Verification items for the finished model (mm, model axes). Face numbers are marked on the shaded views. A direction names the side the tool comes from. Round coordinates to 2 decimals unless told otherwise and drop trailing zeros. Write each loop counter-clockwise with the first axis right and the second up, starting at its lowest first coordinate (ties: lowest second). Pieces come first, ordered by that corner, then holes. Notation, with made-up numbers: (9.25, 83.5) - (44.25, 83.5) arc R19 ccw to (44.25, 110.5) - close; hole circle Ø3 at (43.5, 21.25). An arc over 180 degrees is marked (long way). Answer as a JSON object with one key per item and string values.
```python
from build123d import *

# Parameters (mm, degrees)
CROQUIS1_W                 = 132
CROQUIS1_H                 = 68
SALIENTE_EXTRUIR1_DEPTH    = 8
CORTAR_EXTRUIR1_DEPTH      = 8
CROQUIS3_W                 = 6
CROQUIS3_H                 = 5
SALIENTE_EXTRUIR2_DEPTH    = 8
CROQUIS4_R                 = 2
CROQUIS4_R_2               = 1.6
CORTAR_EXTRUIR2_DEPTH      = 85.029980381
CROQUIS5_R                 = 2.05
CORTAR_EXTRUIR3_DEPTH      = 6
CROQUIS6_W                 = 5
CROQUIS6_H                 = 10
SALIENTE_EXTRUIR3_DEPTH    = 10
CORTAR_EXTRUIR4_DEPTH      = 136.614342899
CORTAR_EXTRUIR4_DEPTH_BACK = 136.614342899
CROQUIS7_R                 = 1.55


with BuildPart() as part:
    # Croquis1 → Saliente-Extruir1 (new body)
    with BuildSketch(Plane(origin=(0, 0, 0), x_dir=(1, 0, 0), z_dir=(0, 1, 0))):
        Rectangle(CROQUIS1_W, CROQUIS1_H)
    extrude(amount=SALIENTE_EXTRUIR1_DEPTH)

    # Croquis2 → Cortar-Extruir1 (cut)
    with BuildSketch(Plane(origin=(0, 8, 0), x_dir=(1, 0, 0), z_dir=(0, 1, 0))):
        Polygon((61, 31.000254068), (66, 31.000254068), (66, 34), (58.000254068, 34), align=None)
        Polygon((66.000254073, 23.155254073), (66, 0.506), (63, 0.506), (63, 20.155), align=None)
    extrude(amount=-CORTAR_EXTRUIR1_DEPTH, mode=Mode.SUBTRACT)

    # Croquis3 → Saliente-Extruir2 (add)
    with BuildSketch(Plane(origin=(0, 8, 0), x_dir=(1, 0, 0), z_dir=(0, 1, 0))):
        with Locations((41.000254068, 36.5)):
            Rectangle(CROQUIS3_W, CROQUIS3_H)
        with Locations((7.000254068, 36.5)):
            Rectangle(CROQUIS3_W, CROQUIS3_H)
        Polygon((-66, 34), (-69.000254073, 30.999745927), (-74.000254073, 30.999745927), (-74.000254073, 21.426745927), (-69.000302023, 16.426793878), (-69.000302023, -7.645206122), (-66, -7.645206122), align=None)
    extrude(amount=-SALIENTE_EXTRUIR2_DEPTH)

    # Croquis4 → Cortar-Extruir2 (cut, through all)
    with BuildSketch(Plane(origin=(0, 8, 0), x_dir=(1, 0, 0), z_dir=(0, 1, 0))):
        with Locations(Location((-59.000302023, 7, 0), (0, 0, 270))):
            Circle(CROQUIS4_R)
        with Locations(Location((-41, -24, 0), (0, 0, 270))):
            Circle(CROQUIS4_R_2)
        with Locations(Location((-31, -24, 0), (0, 0, 270))):
            Circle(CROQUIS4_R_2)
        with Locations(Location((-4.000302023, 8, 0), (0, 0, 270))):
            Circle(CROQUIS4_R)
        with Locations(Location((-4, -7.999999997, 0), (0, 0, 270))):
            Circle(CROQUIS4_R)
        with Locations(Location((26, -22, 0), (0, 0, 270))):
            Circle(CROQUIS4_R_2)
        with Locations(Location((36, -22, 0), (0, 0, 270))):
            Circle(CROQUIS4_R_2)
        with Locations(Location((53, 7, 0), (0, 0, 270))):
            Circle(CROQUIS4_R)
    extrude(amount=-CORTAR_EXTRUIR2_DEPTH, mode=Mode.SUBTRACT)

    # Croquis5 → Cortar-Extruir3 (cut)
    with BuildSketch(Plane(origin=(63, 0, 0), x_dir=(0, 0, -1), z_dir=(1, 0, 0))):
        with Locations((6.506, 4)):
            Circle(CROQUIS5_R)
    extrude(amount=-CORTAR_EXTRUIR3_DEPTH, mode=Mode.SUBTRACT)

    # Croquis6 → Saliente-Extruir3 (add)
    with BuildSketch(Plane.XZ):
        with Locations((-59.000254073, -19)):
            Rectangle(CROQUIS6_W, CROQUIS6_H)
        with Locations((-59.000254073, 22)):
            Rectangle(CROQUIS6_W, CROQUIS6_H)
        with Locations((57.999745927, 22)):
            Rectangle(CROQUIS6_W, CROQUIS6_H)
        with Locations((52.999745927, -19)):
            Rectangle(CROQUIS6_W, CROQUIS6_H)
    extrude(amount=SALIENTE_EXTRUIR3_DEPTH)

    # Croquis7 → Cortar-Extruir4 (cut, two sides: drawn at the far end of the back side and taken through both)
    with BuildSketch(Plane(origin=(55.499745927, 0, 0), x_dir=(0, 0, -1), z_dir=(1, 0, 0)).offset(-CORTAR_EXTRUIR4_DEPTH_BACK)):
        with Locations((19, -4)):
            Circle(CROQUIS7_R)
        with Locations((-22, -4)):
            Circle(CROQUIS7_R)
    extrude(amount=CORTAR_EXTRUIR4_DEPTH + CORTAR_EXTRUIR4_DEPTH_BACK, mode=Mode.SUBTRACT)


solid = part.part
```
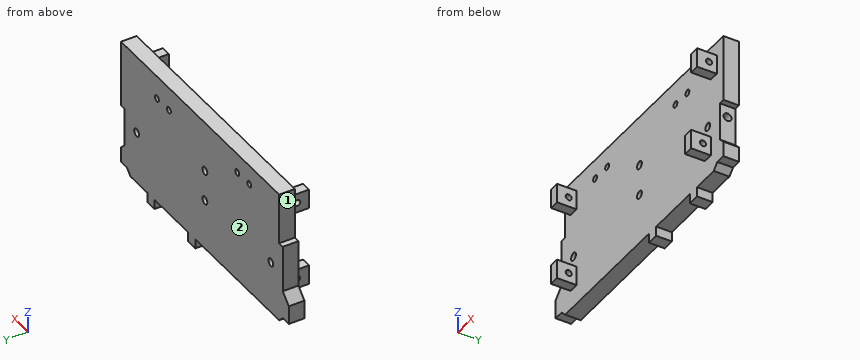
1. Material ranges on probe 1 along Z at (x, y) = (-57.8, -4); probe 2 along X at (y, z) = (5.5, 22); probe 3 along X at (y, z) = (6.25, 24), recorded low to high. Write a range as from..to.
Completed:
{"probe 1": "z = -24..-20.55, -17.45..-14, 17..20.45, 23.55..27", "probe 2": "x = -66..24.4, 27.6..34.4, 37.6..66", "probe 3": "x = -66..-42.6, -39.4..-32.6, -29.4..66"}
2. Cross-section at C-C (x = -64). Record the boundary of the cut face in (y, z), plus the area to 3 significant figures.
Completed:
{"outline": "(0, -34) - (8, -34) - (8, 34) - (0, 34) - close", "area": "544 mm^2"}
3. Cross-section at B-B (x = -41). Record the boundary of the cut face in (y, z), plus the area to 3 significant figures.
Completed:
{"outline": "(0, -34) - (8, -34) - (8, 22.4) - (0, 22.4) - close; (0, 25.6) - (8, 25.6) - (8, 34) - (0, 34) - close", "area": "518 mm^2"}
4. Go/stop test with flat-tipped pins: pin 1 (5.5 mm diameter, centred on x = 53.5, y = -6, fed in from +Z); pin 2 (5 mm diameter, centred on x = -4.5, y = -1, fed in from -Z); pin 3 (5 mm diameter, centred on y = -4, z = -19, fed in from -X). Record where each tip stops, or that it passes through.
Completed:
{"pin 1": "stops at z = 27", "pin 2": "stops at z = -34", "pin 3": "stops at x = -61.5"}
5. Cross-section at A-A (y = -7). Record the boundary of the cut face in (x, z), plus the area to 3 significant figures.
Completed:
{"outline": "(-61.5, -24) - (-56.5, -24) - (-56.5, -14) - (-61.5, -14) - close; (-61.5, 17) - (-56.5, 17) - (-56.5, 27) - (-61.5, 27) - close; (50.5, -24) - (55.5, -24) - (55.5, -14) - (50.5, -14) - close; (55.5, 17) - (60.5, 17) - (60.5, 27) - (55.5, 27) - close", "area": "200 mm^2"}
6. Access from +Z, -Z, +X, -X, +Y, -Y to the whole of each face (thin tool, end or side, straight path). Record for the marked faces 1 and 2.
Completed:
{"face 1": "+Z, -X, +Y, -Y", "face 2": "+Z, -Z, +X, -X, +Y"}
